from build123d import *

# Parameters (mm, degrees)
SKETCH1_W           = 863.6
SKETCH1_H           = 88.9
BOSS_EXTRUDE1_DEPTH = 38.1
SKETCH3_W           = 88.9
SKETCH3_H           = 38.1
CUT_EXTRUDE2_DEPTH  = 39.1
SKETCH4_W           = 88.9
SKETCH4_H           = 19.05
CUT_EXTRUDE3_DEPTH  = 89.9


with BuildPart() as part:
    # Sketch1 → Boss-Extrude1 (new body)
    with BuildSketch(Plane(origin=(0, 0, 0), x_dir=(1, 0, 0), z_dir=(0, 1, 0))):
        with Locations((431.8, 44.45)):
            Rectangle(SKETCH1_W, SKETCH1_H)
    extrude(amount=BOSS_EXTRUDE1_DEPTH)

    # Sketch3 → Cut-Extrude2 (cut, through all)
    with BuildSketch(Plane(origin=(0, 38.1, 0), x_dir=(1, 0, 0), z_dir=(0, 1, 0))):
        with Locations((819.15, 69.85)):
            Rectangle(SKETCH3_W, SKETCH3_H)
    extrude(amount=-CUT_EXTRUDE2_DEPTH, mode=Mode.SUBTRACT)

    # Sketch4 → Cut-Extrude3 (cut, through all)
    with BuildSketch(Plane(origin=(0, 0, -88.9), x_dir=(-1, 0, 0), z_dir=(0, 0, -1))):
        with Locations((-500.0625, 9.525)):
            Rectangle(SKETCH4_W, SKETCH4_H)
    extrude(amount=-CUT_EXTRUDE3_DEPTH, mode=Mode.SUBTRACT)


solid = part.part
Input: part model. Units: mm. Frame: model coordinates. A direction names the side the tool comes from. Coordinates: 2 decimals unless noted, no trailing zeros. Order: outer loops, then holes, each group sorted by start corner. A loop starts at its lowest first (then second) coordinate and runs counter-clockwise, first axis right, second up.
1. Cut plane B-B, the plane z = -22. Return loops of the section in (x, y).
Checked values:
outline: (0, 0) - (455.61, 0) - (455.61, 19.05) - (544.51, 19.05) - (544.51, 0) - (863.6, 0) - (863.6, 38.1) - (0, 38.1) - close
2. Access query for faces 1 (the flat face through (819, 19, -50.8)), 2 (the flat face through (455.612, 9, -45)), 3 (the flat face through (225, 0, -45)). Directions: +Z, -Z, +X, -X, +Y, -Y. A direction counts if a zero-diameter tool reaches every point of the face in a straight line with its end or side. Return the directions, or none.
Checked values:
face 1: -Z, +X, +Y, -Y
face 2: +Z, -Z, -Y
face 3: +Z, -Z, +X, -X, -Y
3. Contact query for a flat-ended pin moving along its axis: P1, Ø3, axis at x = 466.5, z = -15, coming from the -Y side. Output: stop coordinate, or through.
Checked values:
P1: stops at y = 19.05
4. Ray query, line 1 along X through (y, z) = (12.5, -16.5); line 2 along X through (y, z) = (14.5, -66); line 3 along X through (y, z) = (19.5, -69). Return the intervals inside material, ascending.
Checked values:
line 1: x = 0 to 455.61, 544.51 to 863.6
line 2: x = 0 to 455.61, 544.51 to 774.7
line 3: x = 0 to 774.7
5. Draft query along X for faces 4 (the flat face through (544.512, 9, -45)), 5 (the flat face through (426, 19, 0)), 6 (the flat face through (863.6, 19, -25)). Return one class per face: +X half, -X half, draft (parallel to the pull), parting line (faces both ways), or undercut.
Checked values:
face 4: undercut
face 5: draft
face 6: +X half
6. Cut plane C-C, the plane x = 466. Return loops of the section in (y, z), plus the area to 3 significant figures.
Checked values:
outline: (19.05, -88.9) - (38.1, -88.9) - (38.1, 0) - (19.05, 0) - close
area: 1,690 mm2
7. Cut plane D-D, the plane z = -66. Return loops of the section in (x, y), plus the area to 3 significant figures.
Checked values:
outline: (0, 0) - (455.61, 0) - (455.61, 19.05) - (544.51, 19.05) - (544.51, 0) - (774.7, 0) - (774.7, 38.1) - (0, 38.1) - close
area: 27,800 mm2
8. Cut plane A-A, the plane y = 10. Return loops of the section in (x, z).
Checked values:
outline: (0, -88.9) - (455.61, -88.9) - (455.61, 0) - (0, 0) - close; (544.51, -88.9) - (774.7, -88.9) - (774.7, -50.8) - (863.6, -50.8) - (863.6, 0) - (544.51, 0) - close
